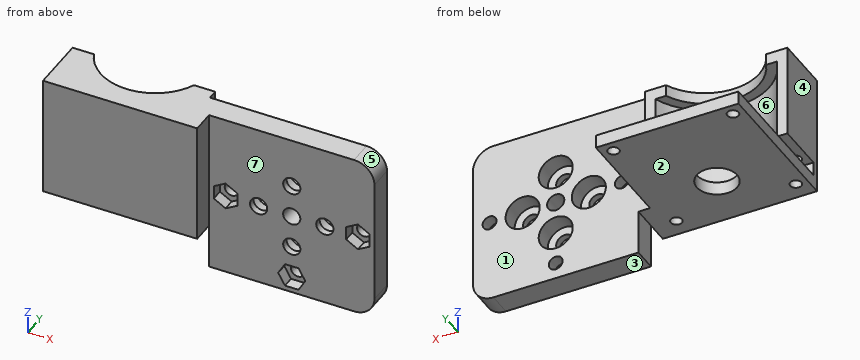
```python
from build123d import *

# Parameters (mm, degrees)
SKETCH_2_W          = 50
SKETCH_2_H          = 50
SKETCH_2_R          = 2.6
EXTRUDE_1_DEPTH     = 2
SKETCH_3_W          = 50
SKETCH_3_H          = 50
SKETCH_3_R          = 5.15
SKETCH_3_R_2        = 2.6
EXTRUDE_2_DEPTH     = 5.2
SKETCH_4_R          = 2.1
CUT_EXTRUDE_1_DEPTH = 10
CUT_EXTRUDE_2_DEPTH = 3.5
FILLET_1_R          = 6.17
FILLET_2_R          = 6.17
SKETCH_7_W          = 43.1
SKETCH_7_H          = 43.1
SKETCH_7_R          = 6.1
SKETCH_7_R_2        = 1.7
EXTRUDE_3_DEPTH     = 4
EXTRUDE_4_DEPTH     = 29
EXTRUDE_5_DEPTH     = 3.5
SKETCH_10_W         = 3.5
SKETCH_10_H         = 11.99
EXTRUDE_6_DEPTH     = 36.5
SKETCH_11_W         = 43.1
SKETCH_11_H         = 43.1
CUT_EXTRUDE_3_DEPTH = 4.2
SKETCH_12_W         = 46.6
SKETCH_12_H         = 36.5
EXTRUDE_7_DEPTH     = 2
SKETCH_13_R         = 1.7
CUT_EXTRUDE_4_DEPTH = 12


with BuildPart() as part:
    # Sketch 2 → Extrude 1 (new body)
    with BuildSketch(Plane(origin=(0, 0, 0), x_dir=(1, 0, 0), z_dir=(0, 1, 0))):
        Rectangle(SKETCH_2_W, SKETCH_2_H)
        Circle(SKETCH_2_R, mode=Mode.SUBTRACT)
        with Locations((10, 0)):
            Circle(SKETCH_2_R, mode=Mode.SUBTRACT)
        with Locations((0, -10)):
            Circle(SKETCH_2_R, mode=Mode.SUBTRACT)
        with Locations((-10, 0)):
            Circle(SKETCH_2_R, mode=Mode.SUBTRACT)
        with Locations((0, 10)):
            Circle(SKETCH_2_R, mode=Mode.SUBTRACT)
    extrude(amount=EXTRUDE_1_DEPTH)

    # Sketch 3 → Extrude 2 (add)
    with BuildSketch(Plane(origin=(0, 2, 0), x_dir=(1, 0, 0), z_dir=(0, 1, 0))):
        Rectangle(SKETCH_3_W, SKETCH_3_H)
        with Locations((0, -10)):
            Circle(SKETCH_3_R, mode=Mode.SUBTRACT)
        with Locations((-10, 0)):
            Circle(SKETCH_3_R, mode=Mode.SUBTRACT)
        Circle(SKETCH_3_R_2, mode=Mode.SUBTRACT)
        with Locations((10, 0)):
            Circle(SKETCH_3_R, mode=Mode.SUBTRACT)
        with Locations((0, 10)):
            Circle(SKETCH_3_R, mode=Mode.SUBTRACT)
    extrude(amount=EXTRUDE_2_DEPTH)

    # Sketch 4 → Cut-Extrude 1 (cut)
    with BuildSketch(Plane(origin=(0, 7.2, 0), x_dir=(1, 0, 0), z_dir=(0, 1, 0))):
        with Locations((20, 0)):
            Circle(SKETCH_4_R)
        with Locations((0, 20)):
            Circle(SKETCH_4_R)
        with Locations((-20, 0)):
            Circle(SKETCH_4_R)
    extrude(amount=-CUT_EXTRUDE_1_DEPTH, mode=Mode.SUBTRACT)

    # Sketch 6 → Cut-Extrude 2 (cut)
    with BuildSketch(Plane.XZ):
        Polygon((-16.45, -2.049593456), (-16.45, 2.049593456), (-20, 4.099186911), (-23.55, 2.049593456), (-23.55, -2.049593456), (-20, -4.099186911), align=None)
        Polygon((2.049593456, -16.45), (-2.049593456, -16.45), (-4.099186911, -20), (-2.049593456, -23.55), (2.049593456, -23.55), (4.099186911, -20), align=None)
        Polygon((16.45, 2.049593456), (16.45, -2.049593456), (20, -4.099186911), (23.55, -2.049593456), (23.55, 2.049593456), (20, 4.099186911), align=None)
    extrude(amount=-CUT_EXTRUDE_2_DEPTH, mode=Mode.SUBTRACT)

    # Fillet 1
    fillet_1_edges = [part.edges().sort_by_distance(p)[0] for p in [
        (25, 3.6, -25),
    ]]
    fillet(fillet_1_edges, radius=FILLET_1_R)

    # Fillet 2
    fillet_2_edges = [part.edges().sort_by_distance(p)[0] for p in [
        (25, 3.6, 25),
    ]]
    fillet(fillet_2_edges, radius=FILLET_2_R)



with BuildPart() as body_2:
    # Sketch 7 → Extrude 3 (new body)
    with BuildSketch(Plane(origin=(0, 0, -11.5), x_dir=(-1, 0, 0), z_dir=(0, 0, -1))):
        with Locations((50.05, 16.76)):
            Rectangle(SKETCH_7_W, SKETCH_7_H)
        with Locations((50.05, 9.71)):
            Circle(SKETCH_7_R, mode=Mode.SUBTRACT)
        with Locations((68.1, 34.81)):
            Circle(SKETCH_7_R_2, mode=Mode.SUBTRACT)
        with Locations((68.1, -1.29)):
            Circle(SKETCH_7_R_2, mode=Mode.SUBTRACT)
        with Locations((32, -1.29)):
            Circle(SKETCH_7_R_2, mode=Mode.SUBTRACT)
        with Locations((32, 34.81)):
            Circle(SKETCH_7_R_2, mode=Mode.SUBTRACT)
    extrude(amount=-EXTRUDE_3_DEPTH)

    # Sketch 8 → Extrude 4 (add)
    with BuildSketch(Plane.XY.offset(-7.5)):
        with BuildLine():
            Line((-71.6, 10.21), (-68.417022078, 10.21))
            ThreePointArc((-68.417022078, 10.21), (-50.05, -2.74), (-31.682977922, 10.21))
            Line((-31.682977922, 10.21), (-28.5, 10.21))
            Line((-28.5, 10.21), (-28.5, -4.79))
            Line((-28.5, -4.79), (-71.6, -4.79))
            Line((-71.6, -4.79), (-71.6, 10.21))
        make_face()
    extrude(amount=EXTRUDE_4_DEPTH)

    # Sketch 9 → Extrude 5 (add)
    with BuildSketch(Plane.XY.offset(21.5)):
        with BuildLine():
            Line((-34.905776679, 10.21), (-28.5, 10.21))
            Line((-28.5, 10.21), (-28.5, -4.79))
            Line((-28.5, -4.79), (-71.6, -4.79))
            Line((-71.6, -4.79), (-71.6, 10.21))
            Line((-71.6, 10.21), (-65.194223321, 10.21))
            ThreePointArc((-65.194223321, 10.21), (-50.05, 0.26), (-34.905776679, 10.21))
        make_face()
    extrude(amount=EXTRUDE_5_DEPTH)


with BuildPart() as part_1:
    add(part.part)

    add(body_2.part)  # Extrude 6 merges body 2
    # Sketch 10 → Extrude 6 (add)
    with BuildSketch(Plane.XY.offset(25)):
        with Locations((-26.75, 1.205)):
            Rectangle(SKETCH_10_W, SKETCH_10_H)
    extrude(amount=-EXTRUDE_6_DEPTH)

    # Sketch 11 → Cut-Extrude 3 (cut)
    with BuildSketch(Plane.XY.offset(-7.5)):
        with Locations((-50.05, 16.76)):
            Rectangle(SKETCH_11_W, SKETCH_11_H)
    extrude(amount=CUT_EXTRUDE_3_DEPTH, mode=Mode.SUBTRACT)

    # Sketch 12 → Extrude 7 (add)
    with BuildSketch(Plane.XZ.offset(4.79)):
        with Locations((-48.3, 6.75)):
            Rectangle(SKETCH_12_W, SKETCH_12_H)
    extrude(amount=EXTRUDE_7_DEPTH)

    # Sketch 13 → Cut-Extrude 4 (cut)
    with BuildSketch(Plane(origin=(0, 0, -11.5), x_dir=(-1, 0, 0), z_dir=(0, 0, -1))):
        with Locations((68.1, 34.81)):
            Circle(SKETCH_13_R)
        with Locations((68.1, -1.29)):
            Circle(SKETCH_13_R)
        with Locations((32, -1.29)):
            Circle(SKETCH_13_R)
        with Locations((32, 34.81)):
            Circle(SKETCH_13_R)
    extrude(amount=-CUT_EXTRUDE_4_DEPTH, mode=Mode.SUBTRACT)


solid = part_1.part
```
Could you check a few things on this model? Use its own coordinates, in mm. Face numbers are marked on the shaded views. A direction names the side the tool comes from. Coordinates: 2 decimals unless noted, no trailing zeros. Write each loop counter-clockwise with the first axis right and the second up, starting at its lowest first coordinate (ties: lowest second). Pieces come first, ordered by that corner, then holes. Notation, with made-up numbers: (-13.5, 53) -> (29.5, 53) arc R25 ccw to (29.5, 72) -> close; hole circle Ø10 at (61, 11.25). An arc over 180 degrees is marked (long way). Write item = value, one per line. Start each with the question number.
(1) I want a section at D-D (x = -10). Please give me the cut outline in (y, z), plus the area to 3 significant figures.
(2) I want a section at B-B (x = 0). Give the number of separate pieces and of enclosed holes in the cut face, plus the area to 3 significant figures.
(3) Will these pins go through, and if not, where does the flat tip stop? pin 1 (6.5 mm diameter, centred on x = -56, y = 4, fed in from -Z); pin 2 (5 mm diameter, centred on x = 0, z = 9.5, fed in from +Y); pin 3 (5 mm diameter, centred on x = -31, z = 10, fed in from +Y).
(4) We'd pull the mould along X, two halves only. Please class the marked faces 4, 5, 6 and 7: released by +X, released by -X, zero draft, split by the parting line, or undercut.
(5) I want a section at C-C (z = 10). Please give me the cut outline in (x, y), plus the area to 3 significant figures.
(6) I want a section at A-A (y = 34.81). Please give me the cut outline in (x, z).
(7) I need wall thicknesses on line 1 (Z direction, x = 0, y = 4.4); line 2 (Z direction, x = 10, y = 0.5); line 3 (Y direction, x = -50.05, z = -8.45). Which ranges of each line are inside material? Lowest first, please. Write a range as [from, to].
(8) Which directions (+Z, -Z, +X, -X, +Y, -Y) give clear straight access to the entire face, cutting with the end or side of a thin tool? Please do the marked faces 1, 2 and 3.
Result set:
q1.outline = (0, -25) -> (7.2, -25) -> (7.2, -5.15) -> (2, -5.15) -> (2, -2.6) -> (0, -2.6) -> close; (0, 2.6) -> (2, 2.6) -> (2, 5.15) -> (7.2, 5.15) -> (7.2, 25) -> (0, 25) -> close
q1.area = 296 mm2
q2.separate_pieces = 5
q2.enclosed_holes = 0
q2.area = 154 mm2
q3.pin_1 = -11.5
q3.pin_2 = 2
q3.pin_3 = 10.21
q4.face_4 = released by -X
q4.face_5 = released by +X
q4.face_6 = undercut
q4.face_7 = zero draft
q5.outline = (-71.6, -6.79) -> (-25, -6.79) -> (-25, 0) -> (-2.6, 0) -> (-2.6, 2) -> (-5.15, 2) -> (-5.15, 7.2) -> (-28.5, 7.2) -> (-28.5, 10.21) -> (-31.68, 10.21) arc R19.5 cw to (-68.42, 10.21) -> (-71.6, 10.21) -> close; (2.6, 0) -> (25, 0) -> (25, 7.2) -> (5.15, 7.2) -> (5.15, 2) -> (2.6, 2) -> close
q5.area = 731 mm2
q6.outline = (-71.6, -11.5) -> (-69.8, -11.5) -> (-69.8, -7.5) -> (-71.6, -7.5) -> close; (-66.4, -11.5) -> (-33.7, -11.5) -> (-33.7, -7.5) -> (-66.4, -7.5) -> close; (-30.3, -11.5) -> (-28.5, -11.5) -> (-28.5, -7.5) -> (-30.3, -7.5) -> close
q7.line_1 = [-25, -22.1], [-17.9, -15.15], [-4.85, -2.6], [2.6, 4.85], [15.15, 25]
q7.line_2 = [-25, -2.6], [2.6, 25]
q7.line_3 = [-6.79, 3.61], [15.81, 38.31]
q8.face_1 = +Z, -Z, +X, +Y
q8.face_2 = -Z, -X, +Y, -Y
q8.face_3 = -Z, +X, -X, +Y, -Y
